For this review, take the finished solid that the model builds, in its own axes (mm). A direction names the side the tool comes from. Give positions to 0.01 mm unless a question says otherwise; leave off trailing zeros. Order: outer loops, then holes, each group sorted by start corner. A loop starts at its lowest first (then second) coordinate and runs counter-clockwise, first axis right, second up.
Item 1: For probe 1 along X at (y, z) = (11.5, 652); probe 2 along Z at (x, y) = (23.75, 14.5), list the stretches that pass through material, from the lowest coordinate up.
Item 2: Consider section C-C (y = 16.5). Give the boundary of the cut face in (x, z), plus the area to 3 significant figures.
Item 3: Consider section A-A (x = 7.5). Give the boundary of the cut face in (y, z), plus the area to 3 significant figures.
Item 4: Machinability: for faces 1 (the flat face through (12, 23.5, 493)), 2 (the flat face through (0, 12, 490)), which of the approach directions +Z, -Z, +X, -X, +Y, -Y give a long, thin tool a straight path to every point of the face, cutting with its end or side? Answer none if there is none.
Item 5: The part is to be moulded in two halves that separate along Y. For faces 3 (the flat face through (1.331, 12.558, 989.932)), 4 (the flat face through (25, 12, 490)), 5 (the flat face through (1.5, 12, 490)), say which applies: released by +Y, released by -Y, zero draft, split by the parting line, or undercut.
Item 6: Consider section B-B (z = 502.5). Give the boundary of the cut face in (x, y), plus the area to 3 significant figures.
Item 7: For P1, Ø12, axis at x = 20, y = 13.5, coming from the +Z side, flat-tipped, find the tip position at first contact; note if it passes through.
```python
from build123d import *

# Parameters (mm, degrees)
SKETCH_W     = 25
SKETCH_H     = 25
SKETCH_W_2   = 22
SKETCH_H_2   = 22
PAD_DEPTH    = 993.5
FILLET_R     = 0.74
POCKET_DEPTH = 25.001


with BuildPart() as part:
    # Sketch → Pad (new body)
    with BuildSketch(Plane.XY):
        with Locations((12.5, 12.5)):
            Rectangle(SKETCH_W, SKETCH_H)
        with Locations((12.5, 12.5)):
            Rectangle(SKETCH_W_2, SKETCH_H_2, mode=Mode.SUBTRACT)
    extrude(amount=PAD_DEPTH)

    # Fillet
    fillet_edges = [part.edges().sort_by_distance(p)[0] for p in [
        (25, 0, 496.75),
        (0, 0, 496.75),
        (25, 25, 496.75),
        (0, 25, 496.75),
    ]]
    fillet(fillet_edges, radius=FILLET_R)

    # Sketch001 (on Face6 of Fillet) → Pocket (cut, through all)
    with BuildSketch(Plane(origin=(0, 0, 0), x_dir=(0, -1, 0), z_dir=(-1, 0, 0))):
        Polygon((0, 0), (-42.302197, 12.12996), (-25.0585, -14.483582), align=None)
        Polygon((-25, 993.5), (23.399026, 979.621803), (15.807791, 1006.485657), align=None)
    extrude(amount=-POCKET_DEPTH, mode=Mode.SUBTRACT)


solid = part.part
```
Resolved:
1. probe 1: x = 0 to 1.5, 23.5 to 25
1. probe 2: z = 4.16 to 990.49
2. outline: (0, 4.73) - (1.5, 4.73) - (1.5, 991.06) - (0, 991.06) - close; (23.5, 4.73) - (25, 4.73) - (25, 991.06) - (23.5, 991.06) - close
2. area: 2,960 mm2
3. outline: (0, 0) - (1.5, 0.43) - (1.5, 986.76) - (0, 986.33) - close; (23.5, 6.74) - (25, 7.17) - (25, 993.5) - (23.5, 993.07) - close
3. area: 2,960 mm2
4. face 1: +Z, -Z
4. face 2: +Z, -Z, -X, +Y, -Y
5. face 3: released by -Y
5. face 4: zero draft
5. face 5: undercut
6. outline: (0, 0.74) arc R0.74 ccw to (0.74, 0) - (24.26, 0) arc R0.74 ccw to (25, 0.74) - (25, 24.26) arc R0.74 ccw to (24.26, 25) - (0.74, 25) arc R0.74 ccw to (0, 24.26) - close; hole (1.5, 1.5) - (23.5, 1.5) - (23.5, 23.5) - (1.5, 23.5) - close
6. area: 141 mm2
7. P1: stops at z = 991.6
